Autodesk Inventor part; units mm, degrees
ref_plane "YZ Plane" through (0, 0, 0) normal (1, 0, 0) x (0, 1, 0)
ref_plane "XZ Plane" through (0, 0, 0) normal (0, 1, 0) x (-1, 0, 0)
ref_plane "XY Plane" through (0, 0, 0) normal (0, 0, 1) x (1, 0, 0)
sketch "Sketch1" plane through (0, 0, 0) normal (0, 1, 0) x (-1, 0, 0)
  circle A0 centre (0, 0) radius 15
  dimension "d0" = 30
extrude "Extrusion1" add sketch "Sketch1" along normal blind 20
sketch "Sketch2" plane through (0, 20, 0) normal (0, 1, 0) x (1, 0, 0)
  circle A0 centre (0, 0) radius 12.5
  dimension "d3" = 25
extrude "Extrusion2" add sketch "Sketch2" along normal blind 25
sketch "Sketch3" plane through (0, 45, 0) normal (0, 1, 0) x (1, 0, 0)
  circle A0 centre (0, 0) radius 6
extrude "Extrusion3" cut sketch "Sketch3" against normal blind 100
sketch "Sketch4" plane through (0, 0, 0) normal (0, -1, 0) x (1, 0, 0)
  circle A0 centre (0, 0) radius 6
  circle A1 centre (0, 0) radius 30
  circle A2 centre (22, 0) radius 4.05
  circle A3 centre (11, 19.0526) radius 4.05
  circle A4 centre (-11, 19.0526) radius 4.05
  circle A5 centre (-22, 0) radius 4.05
  circle A6 centre (-11, -19.0526) radius 4.05
  circle A7 centre (11, -19.0526) radius 4.05
  dimension "d8" = 60
  dimension "d11" = 12
  dimension "d12" = 22
  dimension "d13" = 8.1
  dimension "d16" = 360
extrude "Extrusion4" add sketch "Sketch4" along normal blind 10
sketch "Sketch5" plane through (0, -10, 0) normal (0, -1, 0) x (1, 0, 0)
  circle A0 centre (0, 0) radius 30
  circle A1 centre (11, -19.0526) radius 4.05
  circle A2 centre (-11, -19.0526) radius 4.05
  circle A3 centre (-22, 0) radius 4.05
  circle A4 centre (-11, 19.0526) radius 4.05
  circle A5 centre (11, 19.0526) radius 4.05
  circle A6 centre (22, 0) radius 4.05
  circle A7 centre (0, 0) radius 6
extrude "Extrusion5" add sketch "Sketch5" along normal blind 16.7
properties part number "MiniPodsipnikNatag"
Input: part model. Units: mm. Frame: model coordinates. A direction names the side the tool comes from. Coordinates: 2 decimals unless noted, no trailing zeros. Write each loop counter-clockwise with the first axis right and the second up, starting at its lowest first coordinate (ties: lowest second). Pieces come first, ordered by that corner, then holes. Notation, with made-up numbers: (57.25, -33.75) - (71.25, -33.75) arc R27 cw to (71.25, -3.75) - close; hole circle Ø11 at (-14.5, -35). An arc over 180 degrees is marked (long way). Put each result on its own line as item: value. Start each with the question number.
1) Cut plane D-D (z = -3). Return the cut outline in (x, y), plus the area to 3 significant figures.
2) Mould query, pull axis Z, two halves, no side actions, for faces 3 (the face through (3.4, 20, 12.3)), 4 (the face through (14.985, 9.86, -0.66)), 5 (the face through (17.954, -13.163, -0.178)). Classes: pulls with the +Z half, pulls with the -Z half, needs draft (parallel to the pull), parting line crosses it, or undercut.
3) Reachability of faces 1 (the face through (-3, 45, 5.4)), 2 (the face through (11.923, 32.325, 3.755)) from +Z, -Z, +X, -X, +Y, -Y: full face, straight path, thin tool, end or side. Return the list, or none.
4) Ray query, L1, parallel to Z at x = 0, y = 23; L2, parallel to Z at x = 11, y = -13; L3, parallel to X at y = -10.5, z = 16.5. Return the intervals inside material, ascending.
5) Cut plane C-C (y = -13.5). Return the cut outline in (x, z), plus the area to 3 significant figures.
6) Cut plane B-B (x = 11). Return the cut outline in (y, z), plus the area to 3 significant figures.
7) Cut plane A-A (x = 0). Return the cut outline in (y, z), plus the area to 3 significant figures.
8) Contact query for flat-ended pins moving along their axis: pin 1 (13 mm diameter, centred on x = -22, z = 0, fed in from -Y); pin 2 (1.5 mm diameter, centred on x = -14.5, z = -12.5, fed in from +Y); pin 3 (8 mm diameter, centred on x = -4.5, y = 32.5, fed in from +Z); pin 4 (2 mm diameter, centred on y = 14.5, z = -14.5, fed in from -X). Output: stop coordinate, or through.
Resolved:
1. outline: (-29.85, -26.7) - (-24.72, -26.7) - (-24.72, 0) - (-29.85, 0) - close; (-19.28, -26.7) - (-5.2, -26.7) - (-5.2, 45) - (-12.13, 45) - (-12.13, 20) - (-14.7, 20) - (-14.7, 0) - (-19.28, 0) - close; (5.2, -26.7) - (19.28, -26.7) - (19.28, 0) - (14.7, 0) - (14.7, 20) - (12.13, 20) - (12.13, 45) - (5.2, 45) - close; (24.72, -26.7) - (29.85, -26.7) - (29.85, 0) - (24.72, 0) - close
1. area: 1,750 mm2
2. face 3: needs draft
2. face 4: parting line crosses it
2. face 5: undercut
3. face 1: +Z, -Z, +X, -X, +Y
3. face 2: +Y
4. L1: z = -12.5 to -6, 6 to 12.5
4. L2: z = -27.91 to -23.1, -15 to 15, 23.1 to 27.91
4. L3: x = -25.05 to -14.14, -7.86 to 7.86, 14.14 to 25.05
5. outline: circle Ø60 at (0, 0); hole circle Ø8.1 at (-22, 0); hole circle Ø8.1 at (-11, -19.05); hole circle Ø8.1 at (-11, 19.05); hole circle Ø12 at (0, 0); hole circle Ø8.1 at (11, -19.05); hole circle Ø8.1 at (11, 19.05); hole circle Ø8.1 at (22, 0)
5. area: 2,410 mm2
6. outline: (-26.7, -27.91) - (0, -27.91) - (0, -23.1) - (-26.7, -23.1) - close; (-26.7, -15) - (0, -15) - (0, -10.2) - (20, -10.2) - (20, -5.94) - (45, -5.94) - (45, 5.94) - (20, 5.94) - (20, 10.2) - (0, 10.2) - (0, 15) - (-26.7, 15) - close; (-26.7, 23.1) - (0, 23.1) - (0, 27.91) - (-26.7, 27.91) - close
6. area: 1,760 mm2
7. outline: (-26.7, -30) - (0, -30) - (0, -15) - (20, -15) - (20, -12.5) - (45, -12.5) - (45, -6) - (-26.7, -6) - close; (-26.7, 6) - (45, 6) - (45, 12.5) - (20, 12.5) - (20, 15) - (0, 15) - (0, 30) - (-26.7, 30) - close
7. area: 1,970 mm2
8. pin 1: stops at y = -26.7
8. pin 2: stops at y = 0
8. pin 3: stops at z = 12.49
8. pin 4: stops at x = -6.54
